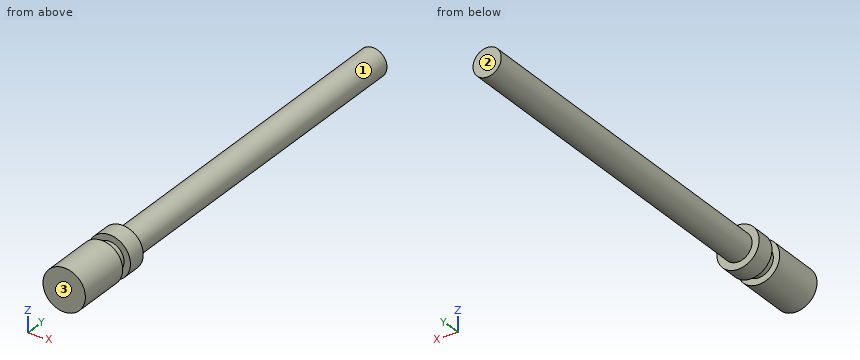
```python
from build123d import *

# Parameters (mm, degrees)
SKETCH_1_R          = 4.5
EXTRUDE_1_DEPTH     = 18
SKETCH_2_R          = 3
EXTRUDE_2_DEPTH     = 96
CUT_EXTRUDE_START   = 11.6
SKETCH_3_OUTSIDE_W  = 30.368
SKETCH_3_OUTSIDE_H  = 30.368
SKETCH_3_OUTSIDE_R  = 3.15
CUT_EXTRUDE_1_DEPTH = 2.4


with BuildPart() as part:
    # 草图1 → 凸台-拉伸1 (new body)
    with BuildSketch(Plane(origin=(0, 0, 0), x_dir=(1, 0, 0), z_dir=(0, 1, 0))):
        with Locations(Location((0, 0, 0), (0, 0, 270))):
            Circle(SKETCH_1_R)
    extrude(amount=EXTRUDE_1_DEPTH)

    # 草图2 → 凸台-拉伸2 (add)
    with BuildSketch(Plane(origin=(0, 0, 0), x_dir=(1, 0, 0), z_dir=(0, 1, 0))):
        with Locations(Location((0, 0, 0), (0, 0, 270))):
            Circle(SKETCH_2_R)
    extrude(amount=EXTRUDE_2_DEPTH)

    # 草图3 outside → 切除-拉伸1 (cut)
    with BuildSketch(Plane(origin=(0, 0, 0), x_dir=(1, 0, 0), z_dir=(0, 1, 0)).offset(CUT_EXTRUDE_START)):
        Rectangle(SKETCH_3_OUTSIDE_W, SKETCH_3_OUTSIDE_H)
        with Locations(Location((0, 0, 0), (0, 0, 270))):
            Circle(SKETCH_3_OUTSIDE_R, mode=Mode.SUBTRACT)
    extrude(amount=CUT_EXTRUDE_1_DEPTH, mode=Mode.SUBTRACT)


solid = part.part
```
Part model, mm, in its own coordinate system. Face numbers are marked on the shaded views. Round coordinates to 2 decimals unless told otherwise and drop trailing zeros. Write each loop counter-clockwise with the first axis right and the second up, starting at its lowest first coordinate (ties: lowest second). Pieces come first, ordered by that corner, then holes. Notation, with made-up numbers: M -37,38 L -27,38 A34 cw -27,72 Z; hole C 72,-9.75 d10. An arc over 180 degrees is marked long. Answer as CSV lines item,"result". Start each with the question number.
1) Drop flat-ended pins along their axis: pin 1 (1.5 mm diameter, centred on x = -1, y = 64, fed in from +Z); pin 2 (3 mm diameter, centred on y = 75.5, z = -1, fed in from +X); pin 3 (2 mm diameter, centred on y = 43, z = -0.5, fed in from -X). Give the stop position or say it passes through.
2) Drill centre lines: L1, parallel to Y at x = 3.75, z = 1.75; L2, parallel to Z at x = 0, y = 36. Where is each one in solid material? Low to high.
3) Mould opens along Y. For the marked faces 1, 2 and 3 say: +Y half, -Y half, draft (parallel to the pull), parting line (faces both ways), or undercut.
4) Band-saw the part on C-C (y = 75). List the corners of the cut face in (x, z), then the cut area to 3 significant figures.
5) Band-saw the part on A-A (z = 0). List the corners of the cut face in (x, y).
6) Band-saw the part on B-B (x = 0). List the corners of the cut face in (y, z), then the cut area to 3 significant figures.
Worked out:
1,pin 1,"z = 2.99"
1,pin 2,"x = 3"
1,pin 3,"x = -3"
2,L1,"0 to 11.6, 14 to 18"
2,L2,"-3 to 3"
3,face 1,"draft"
3,face 2,"+Y half"
3,face 3,"-Y half"
4,outline,"C 0,0 d6"
4,area,"28.3 mm²"
5,outline,"M -4.5,0 L 4.5,0 L 4.5,11.6 L 3.15,11.6 L 3.15,14 L 4.5,14 L 4.5,18 L 3,18 L 3,96 L -3,96 L -3,18 L -4.5,18 L -4.5,14 L -3.15,14 L -3.15,11.6 L -4.5,11.6 Z"
6,outline,"M 0,-4.5 L 11.6,-4.5 L 11.6,-3.15 L 14,-3.15 L 14,-4.5 L 18,-4.5 L 18,-3 L 96,-3 L 96,3 L 18,3 L 18,4.5 L 14,4.5 L 14,3.15 L 11.6,3.15 L 11.6,4.5 L 0,4.5 Z"
6,area,"624 mm²"
